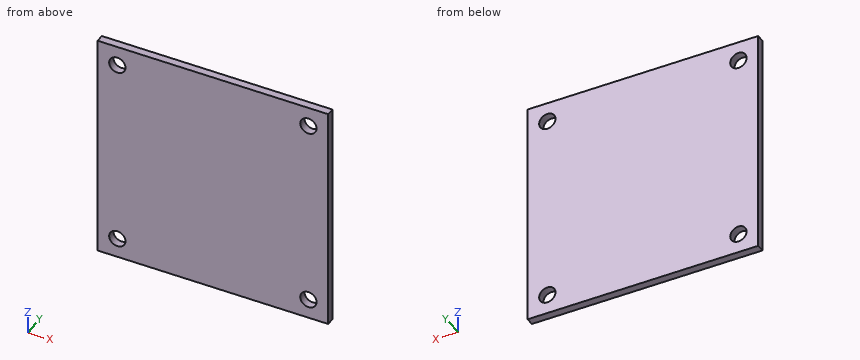
from build123d import *

# Parameters (mm, degrees)
SKETCH1_W               = 46.6
SKETCH1_H               = 46.3
BOSS_EXTRUDE1_DEPTH     = 1.6
SKETCH2_R               = 1.65
CUT_EXTRUDE1_DEPTH      = 46.709051233
MIRROR3_COPY_1_SKETCH_R = 1.65
MIRROR3_COPY_1_DEPTH    = 46.709051233


with BuildPart() as part:
    # Sketch1 → Boss-Extrude1 (new body)
    with BuildSketch(Plane(origin=(0, 0, 0), x_dir=(1, 0, 0), z_dir=(0, 1, 0))):
        with Locations((15.315469417, 1.254976672)):
            Rectangle(SKETCH1_W, SKETCH1_H)
    extrude(amount=BOSS_EXTRUDE1_DEPTH)

    # Sketch2 → Cut-Extrude1 (cut, through all)
    with BuildSketch(Plane.XZ):
        with Locations(Location((-3.984530583, -20.404976672, 0), (0, 0, 270))):
            Circle(SKETCH2_R)
    cut_extrude1 = extrude(amount=-CUT_EXTRUDE1_DEPTH, mode=Mode.SUBTRACT)

    # Mirror1: Cut-Extrude1 across plane
    add(cut_extrude1.mirror(Plane(origin=(15.315469417, 0, 0), x_dir=(0, 0, 1), z_dir=(1, 0, 0))), mode=Mode.SUBTRACT)

    # Mirror3: Cut-Extrude1 across plane
    add(cut_extrude1.mirror(Plane(origin=(0, 0, -1.254976672), x_dir=(1, 0, 0), z_dir=(0, 0, -1))), mode=Mode.SUBTRACT)

    # Mirror3 copy 1 sketch → Mirror3 copy 1 (cut, through all)
    with BuildSketch(Plane(origin=(30.630938834, 0, -2.509953343), x_dir=(-1, 0, 0), z_dir=(0, -1, 0))):
        with Locations(Location((-3.984530583, -20.404976672, 0), (0, 0, 270))):
            Circle(MIRROR3_COPY_1_SKETCH_R)
    extrude(amount=-MIRROR3_COPY_1_DEPTH, mode=Mode.SUBTRACT)


solid = part.part
Source: CAD feature listing. Evaluate the final solid. Frame: model axes, mm. Give positions to 0.01 mm unless a question says otherwise; leave off trailing zeros. Order: outer loops, then holes, each group sorted by start corner. A loop starts at its lowest first (then second) coordinate and runs counter-clockwise, first axis right, second up. Notation, with made-up numbers: (15, 33) -> (25, 33) arc R17 cw to (25, 63) -> close; hole circle Ø9 at (-26, 43). An arc over 180 degrees is marked (long way). Use a Markdown table: item, result.
1) Ray query, line 1 along Z through (x, y) = (34.5, 0.25); line 2 along X through (y, z) = (0.2, -19); line 3 along Z through (x, y) = (34, 1.5). Return the intervals inside material, ascending. Write a range as [from, to].
Answer list:
| item | result |
|---|---|
| line 1 | [-24.4, -22.05], [-18.76, 16.25], [19.54, 21.9] |
| line 2 | [-7.98, -4.85], [-3.12, 33.75], [35.48, 38.62] |
| line 3 | [-24.4, -21.94], [-18.87, 16.36], [19.43, 21.9] |
2) Contact query for flat-ended pins moving along their axis: P1, Ø4, axis at x = -3.98, z = 17.9, coming from the -Y side; P2, Ø2.5, axis at x = -3.98, z = -20.4, coming from the +Y side. Output: stop coordinate, or through.
Answer list:
| item | result |
|---|---|
| P1 | y = 0 |
| P2 | through |
3) Section query A-A, the plane y = 0.8. Return the cut outline in (x, z), then the cut area to 3 significant figures.
Answer list:
| item | result |
|---|---|
| outline | (-7.98, -24.4) -> (38.62, -24.4) -> (38.62, 21.9) -> (-7.98, 21.9) -> close; hole circle Ø3.3 at (-3.98, -20.4); hole circle Ø3.3 at (-3.98, 17.9); hole circle Ø3.3 at (34.62, -20.4); hole circle Ø3.3 at (34.62, 17.9) |
| area | 2,120 mm² |
